from build123d import *

# Parameters (mm, degrees)
F0_R     = 1.778
F0_R_2   = 6.35
F1_DEPTH = 6.35


with BuildPart() as f1:
    # F0 (on Top) → F1 (new body)
    with BuildSketch(Plane.XY):
        Polygon((152.4, 114.3), (-152.4, 114.3), (-152.4, -114.3), (-38.1, -114.3), (-38.1, -158.75), (38.1, -158.75), (38.1, -114.3), (152.4, -114.3), align=None)
        with Locations((-98.679, -60.579)):
            Circle(F0_R, mode=Mode.SUBTRACT)
        with Locations((-88.9, -70.358)):
            Circle(F0_R, mode=Mode.SUBTRACT)
        with BuildLine():
            ThreePointArc((-82.55, -60.579), (-93.390128, -65.069128), (-88.9, -54.229))
            ThreePointArc((-88.9, -54.229), (-84.409872, -56.088872), (-82.55, -60.579))
        make_face(mode=Mode.SUBTRACT)
        with Locations((-79.121, -60.579)):
            Circle(F0_R, mode=Mode.SUBTRACT)
        with Locations((-133.35, -44.958)):
            Circle(F0_R, mode=Mode.SUBTRACT)
        with Locations((-143.129, -35.179)):
            Circle(F0_R, mode=Mode.SUBTRACT)
        with Locations((-133.35, -35.179)):
            Circle(F0_R_2, mode=Mode.SUBTRACT)
        with Locations((-123.571, -35.179)):
            Circle(F0_R, mode=Mode.SUBTRACT)
        with Locations((-133.35, -25.4)):
            Circle(F0_R, mode=Mode.SUBTRACT)
        with BuildLine():
            ThreePointArc((-88.9, -52.578), (-90.157236, -49.542764), (-87.122, -50.8))
            ThreePointArc((-87.122, -50.8), (-87.642764, -52.057236), (-88.9, -52.578))
        make_face(mode=Mode.SUBTRACT)
        with Locations((-98.679, -25.4)):
            Circle(F0_R, mode=Mode.SUBTRACT)
        with Locations((-88.9, -35.179)):
            Circle(F0_R, mode=Mode.SUBTRACT)
        with Locations((-88.9, -25.4)):
            Circle(F0_R_2, mode=Mode.SUBTRACT)
        with Locations((-79.121, -25.4)):
            Circle(F0_R, mode=Mode.SUBTRACT)
        with Locations((66.421, -59.309)):
            Circle(F0_R, mode=Mode.SUBTRACT)
        with Locations((66.421, -25.4)):
            Circle(F0_R, mode=Mode.SUBTRACT)
        with Locations((76.2, -69.088)):
            Circle(F0_R, mode=Mode.SUBTRACT)
        with Locations((76.2, -59.309)):
            Circle(F0_R_2, mode=Mode.SUBTRACT)
        with Locations((85.979, -59.309)):
            Circle(F0_R, mode=Mode.SUBTRACT)
        with Locations((76.2, -49.53)):
            Circle(F0_R, mode=Mode.SUBTRACT)
        with Locations((76.2, -35.179)):
            Circle(F0_R, mode=Mode.SUBTRACT)
        with Locations((76.2, -25.4)):
            Circle(F0_R_2, mode=Mode.SUBTRACT)
        with Locations((85.979, -25.4)):
            Circle(F0_R, mode=Mode.SUBTRACT)
        with Locations((133.35, -44.958)):
            Circle(F0_R, mode=Mode.SUBTRACT)
        with Locations((123.571, -35.179)):
            Circle(F0_R, mode=Mode.SUBTRACT)
        with Locations((133.35, -35.179)):
            Circle(F0_R_2, mode=Mode.SUBTRACT)
        with Locations((143.129, -35.179)):
            Circle(F0_R, mode=Mode.SUBTRACT)
        with Locations((133.35, -25.4)):
            Circle(F0_R, mode=Mode.SUBTRACT)
        with Locations((-88.9, -15.621)):
            Circle(F0_R, mode=Mode.SUBTRACT)
        with Locations((-88.9, 2.921)):
            Circle(F0_R, mode=Mode.SUBTRACT)
        with Locations((-98.679, 12.7)):
            Circle(F0_R, mode=Mode.SUBTRACT)
        with Locations((-88.9, 12.7)):
            Circle(F0_R_2, mode=Mode.SUBTRACT)
        with Locations((-79.121, 12.7)):
            Circle(F0_R, mode=Mode.SUBTRACT)
        with Locations((-88.9, 22.479)):
            Circle(F0_R, mode=Mode.SUBTRACT)
        with Locations((-143.129, 95.25)):
            Circle(F0_R, mode=Mode.SUBTRACT)
        with Locations((-133.35, 85.471)):
            Circle(F0_R, mode=Mode.SUBTRACT)
        with Locations((-133.35, 95.25)):
            Circle(F0_R_2, mode=Mode.SUBTRACT)
        with Locations((-123.571, 95.25)):
            Circle(F0_R, mode=Mode.SUBTRACT)
        with Locations((-133.35, 105.029)):
            Circle(F0_R, mode=Mode.SUBTRACT)
        with Locations((66.421, 12.7)):
            Circle(F0_R, mode=Mode.SUBTRACT)
        with Locations((76.2, -15.621)):
            Circle(F0_R, mode=Mode.SUBTRACT)
        with Locations((76.2, 2.921)):
            Circle(F0_R, mode=Mode.SUBTRACT)
        with Locations((76.2, 12.7)):
            Circle(F0_R_2, mode=Mode.SUBTRACT)
        with Locations((85.979, 12.7)):
            Circle(F0_R, mode=Mode.SUBTRACT)
        with Locations((76.2, 22.479)):
            Circle(F0_R, mode=Mode.SUBTRACT)
        with Locations((123.571, 95.25)):
            Circle(F0_R, mode=Mode.SUBTRACT)
        with Locations((133.35, 85.471)):
            Circle(F0_R, mode=Mode.SUBTRACT)
        with Locations((133.35, 95.25)):
            Circle(F0_R_2, mode=Mode.SUBTRACT)
        with Locations((143.129, 95.25)):
            Circle(F0_R, mode=Mode.SUBTRACT)
        with Locations((133.35, 105.029)):
            Circle(F0_R, mode=Mode.SUBTRACT)
    extrude(amount=F1_DEPTH)


solid = f1.part
Verification items for the finished model (mm, model axes). A direction names the side the tool comes from. Coordinates: 2 decimals unless noted, no trailing zeros. Order: outer loops, then holes, each group sorted by start corner. A loop starts at its lowest first (then second) coordinate and runs counter-clockwise, first axis right, second up. Notation, with made-up numbers: M 77.5,7 L 82.5,7 A23 ccw 82.5,19 Z; hole C -17,12.5 d4. An arc over 180 degrees is marked long. One line per item, written item: value. Start each with the question number.
Item 1: Sectioned sample at A-A (x = -66). Enter the section's corners in (y, z), then the cut area to 3 significant figures.
Item 2: Sectioned sample at B-B (z = 1.5). Count the separate pieces of the cut face and the enclosed holes in it, then the cut area to 3 significant figures.
Item 3: Sectioned sample at C-C (y = -119.5). Enter the section's corners in (x, z).
Item 4: Mould release check, pull along X, two halves, no side actions. Record for faces 4 (the flat face through (-2, -20, 0)), 5 (the cylindrical face through (69.856, -25.121, 3.131)), 6 (the flat face through (-152.4, 2, 3)), 7 (the cylindrical face through (131.973, -41.378, 3.131)): released by +X, released by -X, zero draft, split by the parting line, or undercut.
Item 5: Scan lines: probe 1 along X at (y, z) = (-41, 4); probe 2 along Y at (x, z) = (126.5, 2); probe 3 along X at (y, z) = (-147, 3.5). Record each from-to range of solid material in increasing order.
Item 6: Gauge pin test, flat end, axial feed: pin 1 (1.5 mm diameter, centred on x = -53, z = 1, fed in from -Y). Record the tip position at first contact, or that the pin passes through.
Item 7: Access from +Z, -Z, +X, -X, +Y, -Y to the whole of each face (thin tool, end or side, straight path). Record for faces 1 (the flat face through (94, -114.3, 3)), 2 (the flat face through (-38.1, -136, 3)), 3 (the flat face through (2, 114.3, 3)).
Conclusion:
1. outline: M -114.3,0 L 114.3,0 L 114.3,6.35 L -114.3,6.35 Z
1. area: 1,450 mm^2
2. separate pieces: 1
2. enclosed holes: 50
2. area: 71,400 mm^2
3. outline: M -38.1,0 L 38.1,0 L 38.1,6.35 L -38.1,6.35 Z
4. face 4: zero draft
4. face 5: undercut
4. face 6: released by -X
4. face 7: undercut
5. probe 1: x = -152.4 to -135.89, -130.81 to 130.81, 135.89 to 152.4
5. probe 2: y = -114.3 to 114.3
5. probe 3: x = -38.1 to 38.1
6. pin 1: stops at y = -114.3
7. face 1: +Z, -Z, +X, -Y
7. face 2: +Z, -Z, -X, -Y
7. face 3: +Z, -Z, +X, -X, +Y
